Verification items for the finished model (mm, model axes). A direction names the side the tool comes from. Round coordinates to 2 decimals unless told otherwise and drop trailing zeros. Write each loop counter-clockwise with the first axis right and the second up, starting at its lowest first coordinate (ties: lowest second). Pieces come first, ordered by that corner, then holes. Notation, with made-up numbers: (83.25, 47.25) - (98.25, 47.25) arc R22 cw to (98.25, 63.25) - close; hole circle Ø7 at (9.25, -6.5). An arc over 180 degrees is marked (long way). Answer as a JSON object with one key per item and string values.
```python
from build123d import *

# Parameters (mm, degrees)
SKETCH1_W           = 25.4
SKETCH1_H           = 6.35
BOSS_EXTRUDE1_DEPTH = 127
SKETCH2_R           = 3.96875
CUT_EXTRUDE1_DEPTH  = 77.2


with BuildPart() as part:
    # Sketch1 → Boss-Extrude1 (new body)
    with BuildSketch(Plane(origin=(0, 0, 0), x_dir=(0, 0, -1), z_dir=(1, 0, 0))):
        with Locations((9.890468116, 35.572429457)):
            Rectangle(SKETCH1_W, SKETCH1_H)
        Polygon((28.940468116, 38.747429457), (22.590468116, 38.747429457), (22.590468116, 32.397429457), (22.590468116, -31.102570543), (22.590468116, -37.452570543), (28.940468116, -37.452570543), align=None)
        with Locations((9.890468116, -34.277570543)):
            Rectangle(SKETCH1_W, SKETCH1_H)
    extrude(amount=BOSS_EXTRUDE1_DEPTH)

    # Sketch2 → Cut-Extrude1 (cut, through all)
    with BuildSketch(Plane(origin=(0, 38.747429457, 0), x_dir=(1, 0, 0), z_dir=(0, 1, 0))):
        with Locations((114.3, 9.890468116)):
            Circle(SKETCH2_R)
        with Locations((88.9, 9.890468116)):
            Circle(SKETCH2_R)
        with Locations((63.5, 9.890468116)):
            Circle(SKETCH2_R)
        with Locations((38.1, 9.890468116)):
            Circle(SKETCH2_R)
        with Locations((12.7, 9.890468116)):
            Circle(SKETCH2_R)
    extrude(amount=-CUT_EXTRUDE1_DEPTH, mode=Mode.SUBTRACT)


solid = part.part
```
1. Mould release check, pull along X, two halves, no side actions. Record for faces 1 (the face through (127, 1, -23)), 2 (the face through (0, 1, -23)), 3 (the face through (63, 32.397, -15)), 4 (the face through (9.551, -34.233, -7.476)): released by +X, released by -X, zero draft, split by the parting line, or undercut.
Completed:
{"face 1": "released by +X", "face 2": "released by -X", "face 3": "zero draft", "face 4": "undercut"}
2. Cross-section at C-C (x = 50). Record the boundary of the cut face in (y, z), plus the area to 3 significant figures.
Completed:
{"outline": "(-37.45, -28.94) - (38.75, -28.94) - (38.75, 2.81) - (32.4, 2.81) - (32.4, -22.59) - (-31.1, -22.59) - (-31.1, 2.81) - (-37.45, 2.81) - close", "area": "806 mm^2"}
3. Cross-section at A-A (z = -17). Record the boundary of the cut face in (x, y), plus the area to 3 significant figures.
Completed:
{"outline": "(0, -37.45) - (127, -37.45) - (127, -31.1) - (0, -31.1) - close; (0, 32.4) - (127, 32.4) - (127, 38.75) - (0, 38.75) - close", "area": "1,610 mm^2"}
4. Cross-section at B-B (x = 12.7). Record the boundary of the cut face in (y, z), plus the area to 3 significant figures.
Completed:
{"outline": "(-37.45, -28.94) - (38.75, -28.94) - (38.75, -13.86) - (32.4, -13.86) - (32.4, -22.59) - (-31.1, -22.59) - (-31.1, -13.86) - (-37.45, -13.86) - close; (-37.45, -5.92) - (-31.1, -5.92) - (-31.1, 2.81) - (-37.45, 2.81) - close; (32.4, -5.92) - (38.75, -5.92) - (38.75, 2.81) - (32.4, 2.81) - close", "area": "706 mm^2"}
5. Material ranges on probe 1 along Y at (x, z) = (94.5, -21); probe 2 along Z at (x, y) = (63.5, 37); probe 3 along Z at (x, y) = (100, 23.5), recorded low to high. Write a range as from..to.
Completed:
{"probe 1": "y = -37.45..-31.1, 32.4..38.75", "probe 2": "z = -28.94..-13.86, -5.92..2.81", "probe 3": "z = -28.94..-22.59"}
6. Cross-section at D-D (y = 28.5). Record the boundary of the cut face in (x, z).
Completed:
{"outline": "(0, -28.94) - (127, -28.94) - (127, -22.59) - (0, -22.59) - close"}
7. Access from +Z, -Z, +X, -X, +Y, -Y to the whole of each face (thin tool, end or side, straight path). Record for faces 5 (the face through (63, -31.103, -15)), 6 (the face through (34.951, 35.617, -7.476)).
Completed:
{"face 5": "+Z, +X, -X", "face 6": "+Y, -Y"}
